from build123d import *

# Parameters (mm, degrees)
F1_DEPTH = 25.4
F2_R     = 4.826
F3_DEPTH = 50.801
F5_D     = 9.652
F6_W     = 7.62
F6_H     = 10.16
F7_DEPTH = 62.862793


with BuildPart() as f1:
    # F0 (on Front) → F1 (new body)
    with BuildSketch(Plane.XZ):
        Polygon((-63.5, 50.8), (-101.6, 50.8), (-101.6, 0), (0, 0), (0, 25.4), (-38.1, 25.4), align=None)
    extrude(amount=F1_DEPTH)

    # F2 (on face) → F3 (cut, through all)
    with BuildSketch(Plane.XY.offset(50.8)):
        with Locations((-88.9, -12.7)):
            Circle(F2_R)
    extrude(amount=-F3_DEPTH, mode=Mode.SUBTRACT)

    # F5 (through all)
    with Locations(Plane.XY.offset(25.4)):
        with Locations((-12.7, -12.7)):
            Hole(F5_D / 2)

    # F6 (on face) → F7 (cut, through all)
    with BuildSketch(Plane(origin=(-6.35, 0, -6.35), x_dir=(0.707107, 0, -0.707107), z_dir=(0.707107, 0, 0.707107))):
        with Locations((-64.772308, -12.7)):
            Rectangle(F6_W, F6_H)
    extrude(amount=-F7_DEPTH, mode=Mode.SUBTRACT)


solid = f1.part
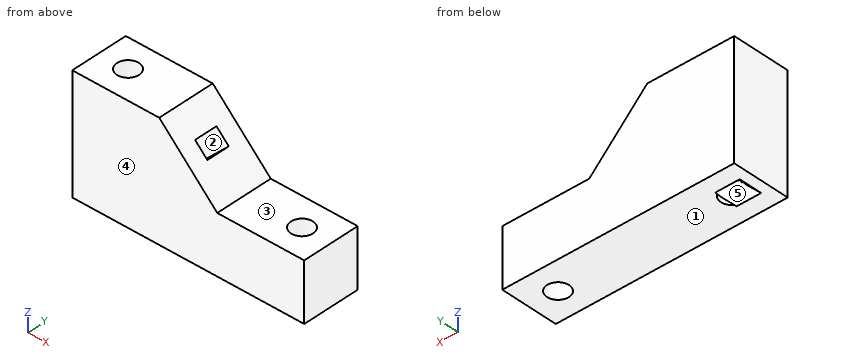
Geometry check sheet. Reference: the model listing, model coordinates, mm. Face numbers are marked on the shaded views. A direction names the side the tool comes from. Round coordinates to 2 decimals unless told otherwise and drop trailing zeros. Loops run counter-clockwise (first coordinate to the right, second up) from the corner with the lowest first, then second, coordinate; pieces in that order, holes last.
Item 1: Thickness scan on line 1 (X direction, y = -15.25, z = 33); line 2 (Y direction, x = -88.9, z = 22.5); line 3 (X direction, y = -12.7, z = 27.5). Record the ranges inside material, lowest first.
Item 2: Cross-section at D-D on z = 29. Record the boundary of the cut face in (x, y).
Item 3: Cross-section at A-A on x = -12.7. Record the boundary of the cut face in (y, z), then the cut area to 3 significant figures.
Item 4: Gauge pin test, flat end, axial feed: pin 1 (3 mm diameter, centred on x = -27.5, y = -18, fed in from +Z). Record the tip position at first contact, or that the pin passes through.
Item 5: Cross-section at B-B on y = -3.5. Record the boundary of the cut face in (x, z).
Item 6: Mould release check, pull along Z, two halves, no side actions. Record for the marked faces 3, 4 and 5: pulls with the +Z half, pulls with the -Z half, needs draft (parallel to the pull), parting line crosses it, or undercut.
Item 7: Cross-section at C-C on z = 38. Record the boundary of the cut face in (x, y), then the cut area to 3 significant figures.
Item 8: Access from +Z, -Z, +X, -X, +Y, -Y to the whole of each face (thin tool, end or side, straight path). Record for the marked faces 1 and 2.
Answer sheet:
1. line 1: x = -101.6 to -93, -84.8 to -63.99, -53.21 to -45.7
1. line 2: y = -25.4 to -17.53, -7.87 to 0
1. line 3: x = -101.6 to -93.73, -84.07 to -69.49, -58.71 to -40.2
2. outline: (-101.6, -25.4) - (-41.7, -25.4) - (-41.7, 0) - (-101.6, 0) - close; hole circle Ø9.65 at (-88.9, -12.7); hole (-67.99, -17.78) - (-57.21, -17.78) - (-57.21, -7.62) - (-67.99, -7.62) - close
3. outline: (-25.4, 0) - (-17.53, 0) - (-17.53, 25.4) - (-25.4, 25.4) - close; (-7.87, 0) - (0, 0) - (0, 25.4) - (-7.87, 25.4) - close
3. area: 400 mm2
4. pin 1: stops at z = 25.4
5. outline: (-101.6, 0) - (0, 0) - (0, 25.4) - (-38.1, 25.4) - (-63.5, 50.8) - (-101.6, 50.8) - close
6. face 3: pulls with the +Z half
6. face 4: needs draft
6. face 5: undercut
7. outline: (-101.6, -25.4) - (-50.7, -25.4) - (-50.7, -17.78) - (-58.99, -17.78) - (-58.99, -7.62) - (-50.7, -7.62) - (-50.7, 0) - (-101.6, 0) - close; hole circle Ø9.65 at (-88.9, -12.7)
7. area: 1,140 mm2
8. face 1: -Z, +X, -X, +Y, -Y
8. face 2: none
